Design review of the part built by this model. Coordinates are the model's own, in mm. A direction names the side the tool comes from. Round coordinates to 2 decimals unless told otherwise and drop trailing zeros. Loops run counter-clockwise (first coordinate to the right, second up) from the corner with the lowest first, then second, coordinate; pieces in that order, holes last. Notation, with made-up numbers: M -12.75,-3.5 L -1.75,-3.5 A27 cw -1.75,24.5 Z; hole C -25.75,24.5 d7. An arc over 180 degrees is marked long. Use a Markdown table: item, result.
from build123d import *

# Parameters (mm, degrees)
F0_R     = 46.0375
F0_R_2   = 43.65625
F1_DEPTH = 50.8
F3_R     = 6.35
F4_DEPTH = 5.588
F6_DEPTH = 92.5205


with BuildPart() as f1:
    # F0 (on Top) → F1 (new body)
    with BuildSketch(Plane.XY):
        Circle(F0_R)
        Circle(F0_R_2, mode=Mode.SUBTRACT)
    extrude(amount=-F1_DEPTH)

    # F3 (on offset) → F4 (cut)
    with BuildSketch(Plane.XZ.offset(46.482)):
        with Locations((0, -50.8)):
            Circle(F3_R)
    extrude(amount=-F4_DEPTH, mode=Mode.SUBTRACT)

    # F5 (on offset) → F6 (cut, through all)
    with BuildSketch(Plane.XZ.offset(46.482)):
        Polygon((-0.034585, -20.435439), (7.456778, -16.150234), (7.491364, -7.51992), (0.034585, -3.174812), (-7.456778, -7.460017), (-7.491364, -16.090331), align=None)
        Polygon((7.456778, -37.105234), (7.491364, -28.47492), (0.034585, -24.129812), (-7.456778, -28.415017), (-7.491364, -37.045331), (-0.034585, -41.390439), align=None)
    extrude(amount=-F6_DEPTH, mode=Mode.SUBTRACT)


solid = f1.part
1. Take a section at C-C on z = -47. Give the boundary of the cut face in (x, y) (1 decimal), and give its area (3 significant figures).
Check values:
| item | result |
|---|---|
| outline | M -5.1,-45.8 L -5.1,-43.4 A43.7 cw long 5.1,-43.4 L 5.1,-45.8 A46 ccw long Z |
| area | 647 mm² |
2. Take a section at A-A on y = 0. Give the boundary of the cut face in (x, z), and give its area (3 significant figures).
Check values:
| item | result |
|---|---|
| outline | M -46.04,-50.8 L -43.66,-50.8 L -43.66,0 L -46.04,0 Z; M 43.66,-50.8 L 46.04,-50.8 L 46.04,0 L 43.66,0 Z |
| area | 242 mm² |
3. Wall thickness on line 1 along X through (y, z) = (0, -28); line 2 along Y through (x, z) = (15.5, -19.5); line 3 along Y through (x, z) = (23.5, -12): over which ranges is each line inside the solid? List them lowest first. Write a range as from..to.
Check values:
| item | result |
|---|---|
| line 1 | x = -46.04..-43.66, 43.66..46.04 |
| line 2 | y = -43.35..-40.81, 40.81..43.35 |
| line 3 | y = -39.59..-36.79, 36.79..39.59 |
4. Machinability: for faces 1 (the face through (-3.82, 44.5, -18.23)), 2 (the face through (-9.46, -42.62, -25.04)), which of the approach directions +Z, -Z, +X, -X, +Y, -Y give a long, thin tool a straight path to every point of the face, cutting with its end or side? Answer none if there is none.
Check values:
| item | result |
|---|---|
| face 1 | +Y, -Y |
| face 2 | +Z, -Z |
5. Insertion check: pin 1 (1 mm diameter, centred on x = -4.5, z = -38.5, fed in from +Y); pin 2 (6 mm diameter, centred on y = -17, z = -33, fed in from +X); pin 3 (1 mm diameter, centred on x = -12, z = -9.5, fed in from +Y). Each pin has a flat end and moves straight along its axis. Give the tip position at first contact, or say it passes through.
Check values:
| item | result |
|---|---|
| pin 1 | stops at y = 45.84 |
| pin 2 | stops at x = 43.86 |
| pin 3 | stops at y = 44.58 |
6. The part is to be moulded in two halves that separate along Z. For faces 3 (the face through (3.815, 44.502, -26.333)), 4 (the face through (0.14, -44.63, -44.45)), say which applies: pulls with the +Z half, pulls with the -Z half, needs draft (parallel to the pull), parting line crosses it, or undercut.
Check values:
| item | result |
|---|---|
| face 3 | undercut |
| face 4 | pulls with the -Z half |
